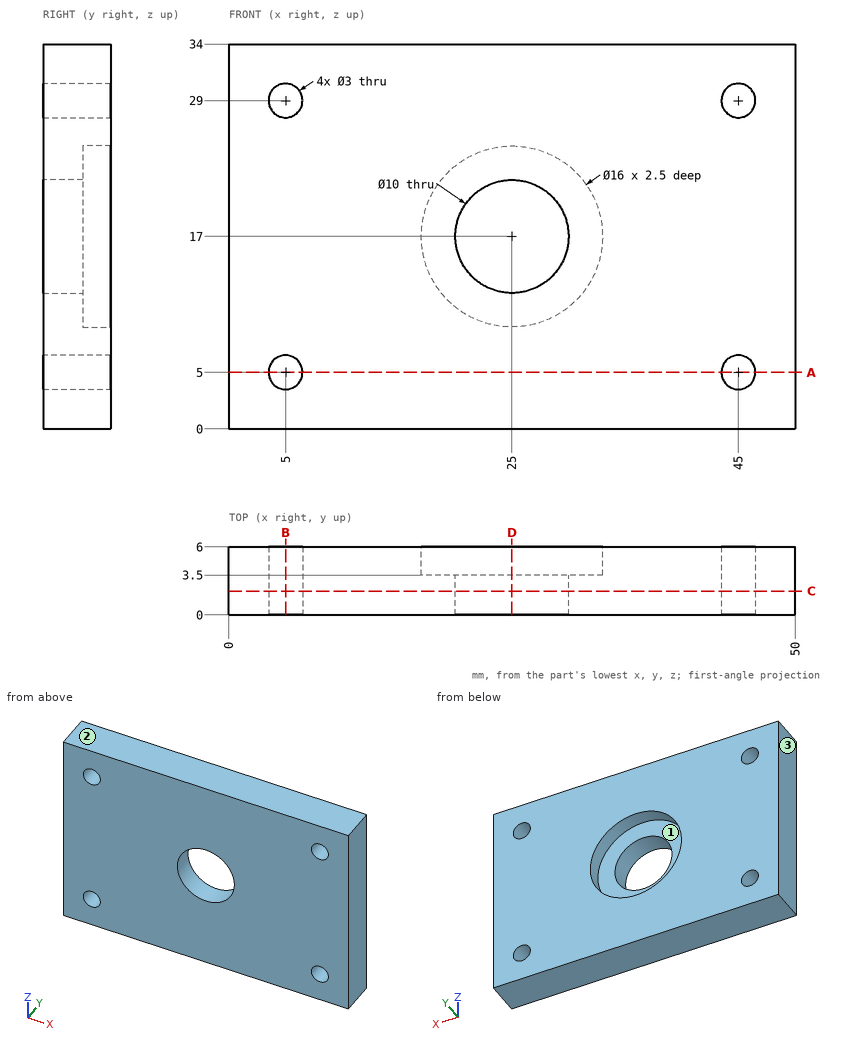
Here's the drawing with two shaded views (mm, measured from the low corner). I have some questions. Coordinates: 2 decimals unless noted, no trailing zeros. Write each loop counter-clockwise with the first axis right and the second up, starting at its lowest first coordinate (ties: lowest second). Pieces come first, ordered by that corner, then holes. Notation, with made-up numbers: (82, 13.5) -> (94, 13.5) arc R8 ccw to (94, 20.5) -> close; hole circle Ø6 at (-32.5, 50). An arc over 180 degrees is marked (long way). One line per question, with ' | ' between items. Start each with the question number.
1. If we section it at D-D (x = 25): Please give me the cut outline in (y, z), and give its area (3 significant figures).
2. Please list where these lines run through material, in increasing order: line 1 along X through (y, z) = (3.25, 5); line 2 along Z through (x, y) = (27, 3.85); line 3 along Z through (x, y) = (29, 5.05).
3. If we section it at A-A (z = 5): Please give me the cut outline in (x, y), and give its area (3 significant figures).
4. If we section it at B-B (x = 5): Please give me the cut outline in (y, z).
5. Will these pins go through, and if not, where does the flat tip stop? P1, Ø1.8, axis at x = 45, z = 29, coming from the +Y side; P2, Ø11.5, axis at x = 25, z = 17, coming from the +Y side.
6. If we section it at C-C (y = 2.1): Please give me the cut outline in (x, z).
7. Thinking about a two-plate mould opening in Z: for the marked faces 1, 2 and 3, which applies, pulls with the +Z half, pulls with the -Z half, needs draft (parallel to the pull), parting line crosses it, or undercut?
Return value:
1) outline: (0, 0) -> (6, 0) -> (6, 9) -> (3.5, 9) -> (3.5, 12) -> (0, 12) -> close; (0, 22) -> (3.5, 22) -> (3.5, 25) -> (6, 25) -> (6, 34) -> (0, 34) -> close | area: 129 mm²
2) line 1: x = 0 to 3.5, 6.5 to 43.5, 46.5 to 50 | line 2: z = 0 to 9.25, 24.75 to 34 | line 3: z = 0 to 10.07, 23.93 to 34
3) outline: (0, 0) -> (3.5, 0) -> (3.5, 6) -> (0, 6) -> close; (6.5, 0) -> (43.5, 0) -> (43.5, 6) -> (6.5, 6) -> close; (46.5, 0) -> (50, 0) -> (50, 6) -> (46.5, 6) -> close | area: 264 mm²
4) outline: (0, 0) -> (6, 0) -> (6, 3.5) -> (0, 3.5) -> close; (0, 6.5) -> (6, 6.5) -> (6, 27.5) -> (0, 27.5) -> close; (0, 30.5) -> (6, 30.5) -> (6, 34) -> (0, 34) -> close
5) P1: passes through | P2: stops at y = 3.5
6) outline: (0, 0) -> (50, 0) -> (50, 34) -> (0, 34) -> close; hole circle Ø3 at (5, 5); hole circle Ø3 at (5, 29); hole circle Ø10 at (25, 17); hole circle Ø3 at (45, 5); hole circle Ø3 at (45, 29)
7) face 1: undercut | face 2: pulls with the +Z half | face 3: needs draft
